Input: part model. Units: mm. Frame: model coordinates. A direction names the side the tool comes from. Round coordinates to 2 decimals unless told otherwise and drop trailing zeros. Loops run counter-clockwise (first coordinate to the right, second up) from the corner with the lowest first, then second, coordinate; pieces in that order, holes last. Notation, with made-up numbers: M 18.25,22 L 67.25,22 A7 cw 67.25,35 Z; hole C 82.5,-5 d9. An arc over 180 degrees is marked long. Return JSON: item names as keys, results as strings. Group by question number.
1) Section B-B (x = 0). Output: boundary loops of the cut face in (y, z), plus the area to 3 significant figures.
2) Material intervals for line 1 (Y direction, x = 28.05, z = -26); line 2 (X direction, y = 103, z = -17.5); line 3 (X direction, y = -7.59, z = 0.9), sorted ascending. Write a range as from..to.
3) Section C-C (y = 80). Output: boundary loops of the cut face in (x, z), plus the area to 3 significant figures.
4) Contact query for flat-ended pins moving along their axis: P1, Ø4.5, axis at x = -26.5, z = -13.5, coming from the -Y side; P2, Ø1, axis at x = 7, y = 73.5, coming from the -Z side; P3, Ø5.5, axis at x = 13.15, y = -7.59, coming from the +Z side. Output: stop coordinate, or through.
5) Access query for faces 4 (the face through (27.986, 78.414, -25.792)), 5 (the face through (0, 44, 0)). Directions: +Z, -Z, +X, -X, +Y, -Y. A direction counts if a zero-diameter tool reaches every point of the face in a straight line with its end or side. Return the directions, or none.
6) Section D-D (z = -10). Output: boundary loops of the cut face in (x, y), plus the area to 3 significant figures.
7) Section A-A (z = -26). Output: boundary loops of the cut face in (x, y), plus the area to 3 significant figures.
8) Mould query, pull axis X, two halves, no side actions, for faces 1 (the face through (0.509, -23.494, 0.986)), 2 (the face through (27.986, 98.414, -25.792)), 3 (the face through (27, 85, -19)). Classes: +X half, -X half, draft (parallel to the pull), parting line (faces both ways), or undercut.
Autodesk Inventor part; units mm, degrees
ref_plane "YZ Plane" through (0, 0, 0) normal (1, 0, 0) x (0, 1, 0)
ref_plane "XZ Plane" through (0, 0, 0) normal (0, 1, 0) x (-1, 0, 0)
ref_plane "XY Plane" through (0, 0, 0) normal (0, 0, 1) x (1, 0, 0)
sketch "スケッチ1" plane through (0, 0, 0) normal (0, 0, 1) x (1, 0, 0)
  circle A0 centre (0, 0) radius 23.5
  line L0 (0, 0) -> (0, 60)
  line L1 (0, 60) -> (25, 60)
  line L2 (25, 60) -> (25, 110)
  line L3 (25, 110) -> (0, 110)
  line L4 (0, 110) -> (0, 60)
  line L5 (25, 60) -> (23.4927, -0.5845)
  line L6 (0, 60) -> (-25, 60)
  line L7 (-25, 60) -> (-25, 110)
  line L8 (-25, 110) -> (0, 110)
  line L9 (-25, 60) -> (-23.4927, -0.5845)
  point P0 (-23.4927, -0.5845)
  dimension "d0" = 47
  dimension "d1" = 60
  dimension "d2" = 50
  dimension "d3" = 25
extrude "プレート1" add sketch "スケッチ1" along normal blind 2
sketch "スケッチ2" plane through (27, 60, -2) normal (1, 0, 0) x (0, 1, 0)
  line L0 (50, 0) -> (0, 0)
  line L1 (0, 0) -> (0, -34)
  line L2 (0, -34) -> (50, -34)
  line L3 (50, -34) -> (50, 0)
edge flange "フランジ1" height 38 angle 90 thickness 2 bend radius 2 thickness toward (1, 0, 0) relief tear relief width 2 relief depth 1 edges at (25, 85, 0) wall of the first edge with corners at (27, 110, -2) (27, 60, -2) (27, 60, -36) (27, 110, -36)
bend "曲げ1"
corner "コーナー1"
sketch "スケッチ3" plane through (-27, 110, -2) normal (-1, 0, 0) x (0, -1, 0)
  line L0 (50, 0) -> (0, 0)
  line L1 (0, 0) -> (0, -34)
  line L2 (0, -34) -> (50, -34)
  line L3 (50, -34) -> (50, 0)
edge flange "フランジ2" height 38 angle 90 thickness 2 bend radius 2 thickness toward (-1, 0, 0) relief tear relief width 2 relief depth 1 edges at (-25, 85, 0) wall of the first edge with corners at (-27, 60, -2) (-27, 110, -2) (-27, 110, -36) (-27, 60, -36)
bend "曲げ2"
corner "コーナー2"
sketch "スケッチ4" plane through (0, 0, 2) normal (0, 0, 1) x (1, 0, 0)
  circle A0 centre (0, 0) radius 10.1
  dimension "d25" = 20.2
extrude "押し出し1" cut sketch "スケッチ4" against normal blind 10
sketch "スケッチ5" plane through (0, 0, 2) normal (0, 0, 1) x (1, 0, 0)
  circle A0 centre (0, 0) radius 15.18
  point P0 (0, 15.18)
  point P1 (-13.1463, 7.59)
  point P2 (-13.1463, -7.59)
  point P3 (0, -15.18)
  point P4 (13.1463, -7.59)
  point P5 (13.1463, 7.59)
  dimension "d28" = 30.36
  dimension "d31" = 360
hole "穴1" at (0, 15.18, 2) at (-13.1463, 7.59, 2) at (-13.1463, -7.59, 2) at (0, -15.18, 2) at (13.1463, -7.59, 2) at (13.1463, 7.59, 2) direction (0, 0, -1) diameter 4.1 end through all
sketch "スケッチ6" plane through (29, 60, -36) normal (1, 0, 0) x (0, 0, -1)
  line L0 (0, 0) -> (0, 50)
  line L1 (0, 10) -> (-34, 10)
  line L2 (-34, 50) -> (-34, 0)
  line L3 (0, 0) -> (-34, 0)
  line L4 (0, 50) -> (-34, 50)
  line L5 (-10, 50) -> (-10, 10)
  point P0 (-36, -60)
  point P1 (-10, 20)
  point P2 (-10, 40)
  point P3 (-36, 50)
  dimension "d40" = 10
  dimension "d42" = 10
  dimension "d43" = 20
  dimension "d62" = 26
hole "穴2" at (29, 80, -26) at (29, 100, -26) direction (-1, 0, 0) diameter 3.2 end through all
sketch "スケッチ7" plane through (0, 0, 2) normal (0, 0, 1) x (1, 0, 0)
  line L0 (-15, 100) -> (15, 100)
  line L1 (15, 100) -> (15, 60)
  line L2 (15, 60) -> (-15, 60)
  line L3 (-15, 60) -> (-15, 100)
  line L4 (-25, 110) -> (25, 110)
  line L5 (-25, 60) -> (-25, 110)
  line L6 (25, 110) -> (25, 60)
  circle A0 centre (0, 0) radius 10.1
  circle A1 centre (0, 0) radius 13.5
  line L7 (-13.4958, -0.3358) -> (-14.7481, 50)
  line L8 (-23.4927, -0.5845) -> (-25, 60)
  line L9 (13.4958, -0.3358) -> (14.7481, 50)
  line L10 (25, 60) -> (23.4927, -0.5845)
  line L11 (-14.7481, 50) -> (14.7481, 50)
  line L12 (-14.0018, 20) -> (14.0018, 20)
  dimension "d51" = 10
  dimension "d52" = 10
  dimension "d53" = 10
  dimension "d54" = 40
  dimension "d55" = 10
  dimension "d56" = 10
  dimension "d57" = 20
extrude "押し出し2" [suppressed]
fillet "フィレット1" [suppressed]
fillet "フィレット2" radius 2 4 edges at (-28, 60, -36) (-28, 110, -36) (28, 60, -36) (28, 110, -36)
equation "\"d38\" = Thickness"
equation "\"d4\" = Thickness"
equation "\"d5\" = BendReliefWidth"
equation "\"d6\" = BendReliefDepth"
equation "\"d7\" = MinimumRemnant"
equation "\"d8\" = TransitionRadius"
equation "\"d11\" = BendRadius"
equation "\"d12\" = CornerReliefSize"
equation "\"d13\" = GapSize"
equation "\"d14\" = JacobiRadiusSize"
equation "\"d15\" = BendReliefWidth"
equation "\"d16\" = BendReliefDepth"
equation "\"d17\" = MinimumRemnant"
equation "\"d18\" = TransitionRadius"
equation "\"d21\" = BendRadius"
equation "\"d22\" = CornerReliefSize"
equation "\"d23\" = GapSize"
equation "\"d24\" = JacobiRadiusSize"
equation "\"BendRadius\" = Thickness"
equation "\"BendReliefWidth\" = Thickness"
equation "\"BendReliefDepth\" = 0.5 * Thickness"
equation "\"CornerReliefSize\" = 4 * Thickness"
equation "\"MinimumRemnant\" = 2 * Thickness"
equation "\"TransitionRadius\" = BendRadius"
equation "\"JacobiRadiusSize\" = BendRadius"
equation "\"GapSize\" = Thickness"
properties part number "servoplate1_forR3" material "アルミニウム 6061"
Returned:
{
 "1": {"outline": "M -23.5,0 L -17.23,0 L -17.23,2 L -23.5,2 Z; M -13.13,0 L -10.1,0 L -10.1,2 L -13.13,2 Z; M 10.1,0 L 13.13,0 L 13.13,2 L 10.1,2 Z; M 17.23,0 L 110,0 L 110,2 L 17.23,2 Z", "area": "210 mm^2"},
 "2": {"line 1": "y = 60..78.4, 81.6..98.4, 101.6..110", "line 2": "x = -29..-27, 27..29", "line 3": "x = -22.24..-15.2, -11.1..-6.66, 6.66..11.1, 15.2..22.24"},
 "3": {"outline": "M -29,-36 L -27,-36 L -27,-27.6 L -29,-27.6 Z; M -29,-24.4 L -27,-24.4 L -27,-2 A2 cw -25,0 L 25,0 A2 cw 27,-2 L 27,-24.4 L 29,-24.4 L 29,-2 A4 ccw 25,2 L -25,2 A4 ccw -29,-2 Z; M 27,-36 L 29,-36 L 29,-27.6 L 27,-27.6 Z", "area": "242 mm^2"},
 "4": {"P1": "stops at y = 60", "P2": "stops at z = 0", "P3": "stops at z = 2"},
 "5": {"face 4": "+X, -X", "face 5": "-Z, +Y, -Y"},
 "6": {"outline": "M -29,60 L -27,60 L -27,110 L -29,110 Z; M 27,60 L 29,60 L 29,110 L 27,110 Z", "area": "200 mm^2"},
 "7": {"outline": "M -29,60 L -27,60 L -27,78.4 L -29,78.4 Z; M -29,81.6 L -27,81.6 L -27,98.4 L -29,98.4 Z; M -29,101.6 L -27,101.6 L -27,110 L -29,110 Z; M 27,60 L 29,60 L 29,78.4 L 27,78.4 Z; M 27,81.6 L 29,81.6 L 29,98.4 L 27,98.4 Z; M 27,101.6 L 29,101.6 L 29,110 L 27,110 Z", "area": "174 mm^2"},
 "8": {"face 1": "parting line", "face 2": "draft", "face 3": "undercut"}
}
